Autodesk Inventor part; units mm, degrees
ref_plane "YZ Plane" through (0, 0, 0) normal (1, 0, 0) x (0, 1, 0)
ref_plane "XZ Plane" through (0, 0, 0) normal (0, 1, 0) x (-1, 0, 0)
ref_plane "XY Plane" through (0, 0, 0) normal (0, 0, 1) x (1, 0, 0)
sketch "Esboço1" plane through (0, 0, 0) normal (0, 0, 1) x (1, 0, 0)
  line L0 (0, 0) -> (40.5, 0)
  line L1 (40.5, 0) -> (40.5, 27.5)
  line L2 (40.5, 27.5) -> (0, 27.5)
  line L3 (0, 27.5) -> (0, 0)
  line L4 (15, 20.75) -> (10, 20.75)
  line L5 (10, 20.75) -> (10, 6.75)
  line L6 (10, 6.75) -> (15, 6.75)
  line L7 (15, 6.75) -> (20, 6.75)
  line L8 (20, 6.75) -> (20, 20.75)
  line L9 (20, 20.75) -> (15, 20.75)
  line L10 (40.5, 27.5) -> (40.5, 22.5)
  line L11 (40.5, 22.5) -> (35.5, 22.5)
  line L12 (40.5, 0) -> (40.5, 5)
  line L13 (40.5, 5) -> (35.5, 5)
  line L14 (0, 0) -> (0, 5)
  line L15 (0, 5) -> (5, 5)
  line L16 (0, 27.5) -> (0, 22.5)
  line L17 (0, 22.5) -> (5, 22.5)
  circle A0 centre (5, 22.5) radius 1.5
  circle A1 centre (5, 5) radius 1.5
  circle A2 centre (35.5, 22.5) radius 1.5
  circle A3 centre (35.5, 5) radius 1.5
  dimension "d0" = 40.5
  dimension "d1" = 27.5
  dimension "d5" = 5
  dimension "d6" = 5
  dimension "d7" = 5
  dimension "d8" = 5
  dimension "d9" = 5
  dimension "d10" = 5
  dimension "d11" = 5
  dimension "d12" = 5
  dimension "d13" = 5
  dimension "d14" = 5
  dimension "d15" = 3
  dimension "d16" = 3
  dimension "d17" = 3
  dimension "d18" = 3
extrude "Extrusão1" add sketch "Esboço1" along normal blind 2 contours L3 L2 L1 L0 | L9 L8 L7 L6 L5 L4
fillet "Arredondamento1" radius 2 4 edges at (0, 27.5, 1) (0, 0, 1) (40.5, 27.5, 1) (40.5, 0, 1)
extrude "Extrusão2" add sketch "Esboço1" along normal blind 7 contours L9 L8 L7 L6 L5 L4
extrude "Extrusão3" add sketch "Esboço1" along normal blind 2 contours A3 | A2 | A0 | A1
properties part number "CASE ESP32 CAM - Tampa"
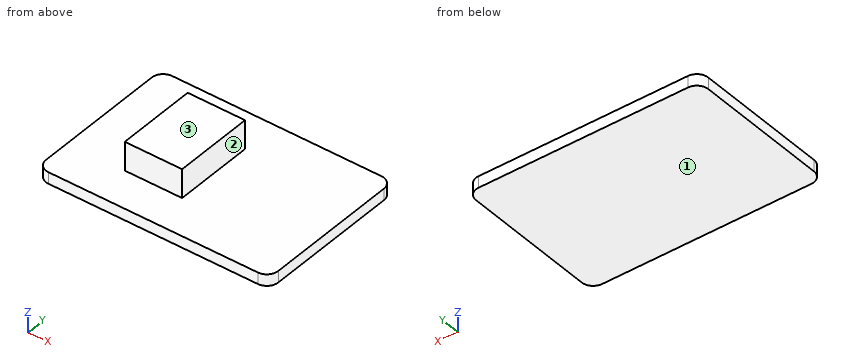
Read the model definition and answer for the solid it produces. Units are mm, in the model's axes. Face numbers are marked on the shaded views. Give positions to 0.01 mm unless a question says otherwise; leave off trailing zeros. Write each loop counter-clockwise with the first axis right and the second up, starting at its lowest first coordinate (ties: lowest second). Pieces come first, ordered by that corner, then holes. Notation, with made-up numbers: M -15,-1.75 L 38,-1.75 A22 ccw 38,31.25 Z; hole C 59,-0.75 d11. An arc over 180 degrees is marked long. Put each result on its own line as item: value. Start each with the question number.
1. The part is cut by section B-B, the plane y = 12. Give the vertices of the cut face in (x, z).
2. For a pull along Z with two mould halves and no side action, classify the marked faces 1, 2 and 3 as released by +Z, released by -Z, zero draft, split by the parting line, or undercut.
3. Each of these flat-tipped pins is pushed along its axis until it touches: pin 1 Ø1.5 at (x, z) = (13, 5.5) entering from -Y; pin 2 Ø2 at (x, y) = (6.5, 10.5) entering from +Z; pin 3 Ø2.5 at (y, z) = (15, 5.5) entering from +X. Where does it stop, or does it pass through?
4. The part is cut by section A-A, the plane x = 17. Give the vertices of the cut face in (y, z).
5. The part is cut by section D-D, the plane y = 22. Give the vertices of the cut face in (x, z).
6. Consider line 1 along Y through (x, z) = (19, 6.25); line 2 along Z through (x, y) = (27.5, 25.25); line 3 along X through (y, z) = (13.75, 6.75). Determine where each line is inside the solid, lowest interval first.
7. The part is cut by section C-C, the plane z = 4.75. Give the vertices of the cut face in (x, y), and give its area (3 significant figures).
Final values:
1. outline: M 0,0 L 40.5,0 L 40.5,2 L 20,2 L 20,7 L 10,7 L 10,2 L 0,2 Z
2. face 1: released by -Z
2. face 2: zero draft
2. face 3: released by +Z
3. pin 1: stops at y = 6.75
3. pin 2: stops at z = 2
3. pin 3: stops at x = 20
4. outline: M 0,0 L 27.5,0 L 27.5,2 L 20.75,2 L 20.75,7 L 6.75,7 L 6.75,2 L 0,2 Z
5. outline: M 0,0 L 40.5,0 L 40.5,2 L 0,2 Z
6. line 1: y = 6.75 to 20.75
6. line 2: z = 0 to 2
6. line 3: x = 10 to 20
7. outline: M 10,6.75 L 20,6.75 L 20,20.75 L 10,20.75 Z
7. area: 140 mm²
